Part model, mm, in its own coordinate system. Give positions to 0.01 mm unless a question says otherwise; leave off trailing zeros.
1. Slice it at A-A on y = -1.9. Give the number of separate pieces and of enclosed holes in the cut face, and give its area (3 significant figures).
2. Probe line 1 (Z direction, x = 42, y = -2.9); line 2 (Z direction, x = -129, y = -0.95); line 3 (X direction, y = -2.25, z = -5.5). List the from-to ranges inside material, lowest first.
3. Drop flat-ended pins along their axis: pin 1 Ø2.5 at (x, z) = (-88, 1) entering from -Y; pin 2 Ø1 at (y, z) = (-2.5, -1.5) entering from +X. Give the stop position or say it passes through.
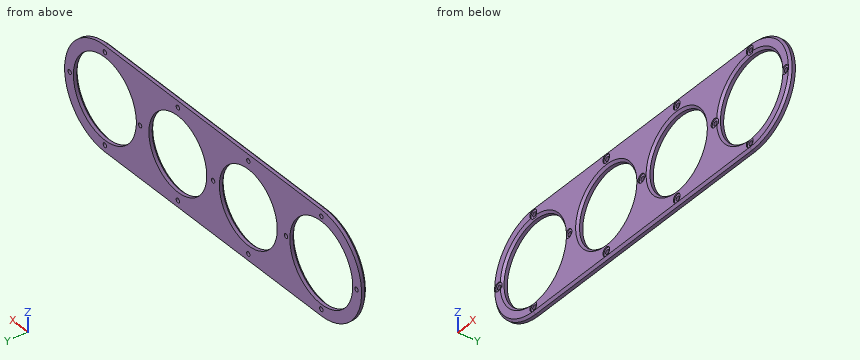
from build123d import *

# Parameters (mm, degrees)
F0_R     = 2
F0_R_2   = 37.5
F0_R_3   = 34.5
F1_DEPTH = 5
F2_SIZE  = 2
F3_SIZE  = 2
F4_R     = 4
F5_DEPTH = 1
F6_SIZE  = 1.99999


# Not quite as in the source:
# - a fillet or chamfer is up to 0.001 mm smaller than in the source, because OpenCascade refuses the exact size


with BuildPart() as f1:
    # F0 (on Front) → F1 (new body)
    with BuildSketch(Plane.XZ):
        with BuildLine():
            ThreePointArc((129, -48), (177, 0), (129, 48))
            Line((129, 48), (0, 48))
            Line((0, 48), (-129, 48))
            ThreePointArc((-129, 48), (-177, 0), (-129, -48))
            Line((-129, -48), (0, -48))
            Line((0, -48), (129, -48))
        make_face()
        with Locations((-129, -42)):
            Circle(F0_R, mode=Mode.SUBTRACT)
        with Locations((-42, -42)):
            Circle(F0_R, mode=Mode.SUBTRACT)
        with Locations((42, -42)):
            Circle(F0_R, mode=Mode.SUBTRACT)
        with Locations((129, -42)):
            Circle(F0_R, mode=Mode.SUBTRACT)
        with Locations((-171, 0)):
            Circle(F0_R, mode=Mode.SUBTRACT)
        with Locations((-129, 0)):
            Circle(F0_R_2, mode=Mode.SUBTRACT)
        with Locations((-87, 0)):
            Circle(F0_R, mode=Mode.SUBTRACT)
        with Locations((-42, 0)):
            Circle(F0_R_3, mode=Mode.SUBTRACT)
        with Locations((-129, 42)):
            Circle(F0_R, mode=Mode.SUBTRACT)
        with Locations((-42, 42)):
            Circle(F0_R, mode=Mode.SUBTRACT)
        Circle(F0_R, mode=Mode.SUBTRACT)
        with Locations((42, 0)):
            Circle(F0_R_3, mode=Mode.SUBTRACT)
        with Locations((87, 0)):
            Circle(F0_R, mode=Mode.SUBTRACT)
        with Locations((129, 0)):
            Circle(F0_R_2, mode=Mode.SUBTRACT)
        with Locations((171, 0)):
            Circle(F0_R, mode=Mode.SUBTRACT)
        with Locations((42, 42)):
            Circle(F0_R, mode=Mode.SUBTRACT)
        with Locations((129, 42)):
            Circle(F0_R, mode=Mode.SUBTRACT)
    extrude(amount=F1_DEPTH)

    # F2
    f2_edges = [f1.edges().sort_by_distance(p)[0] for p in [
        (7.5, -5, 0),
        (-76.5, -5, 0),
    ]]
    chamfer(f2_edges, length=F2_SIZE)

    # F3
    f3_edges = [f1.edges().sort_by_distance(p)[0] for p in [
        (91.5, -5, 0),
        (-166.5, -5, 0),
    ]]
    chamfer(f3_edges, length=F3_SIZE)

    # F4 (on face) → F5 (cut)
    with BuildSketch(Plane.XZ.offset(5)):
        Circle(F4_R)
        with Locations((42, 42)):
            Circle(F4_R)
        with Locations((42, -42)):
            Circle(F4_R)
        with Locations((129, 42)):
            Circle(F4_R)
        with Locations((87, 0)):
            Circle(F4_R)
        with Locations((129, -42)):
            Circle(F4_R)
        with Locations((171, 0)):
            Circle(F4_R)
        with Locations((-42, 42)):
            Circle(F4_R)
        with Locations((-42, -42)):
            Circle(F4_R)
        with Locations((-87, 0)):
            Circle(F4_R)
        with Locations((-129, -42)):
            Circle(F4_R)
        with Locations((-129, 42)):
            Circle(F4_R)
        with Locations((-171, 0)):
            Circle(F4_R)
    extrude(amount=-F5_DEPTH, mode=Mode.SUBTRACT)

    # F6 (size 2 in the source; OpenCascade refuses exactly that, so slightly less here)
    f6_edges = [f1.edges().sort_by_distance(p)[0] for p in [
        (-177, -5, 0),
        (0, -5, 48),
        (0, -5, -48),
        (177, -5, 0),
    ]]
    chamfer(f6_edges, length=F6_SIZE)


solid = f1.part
Data:
1. separate pieces: 1
1. enclosed holes: 17
1. area: 15,500 mm2
2. line 1: z = -48 to -44, -40 to -34.5, 34.5 to 40, 44 to 48
2. line 2: z = -48 to -44, -40 to -37.5, 37.5 to 40, 44 to 48
2. line 3: x = -176.68 to -166.09, -91.91 to -76.06, -7.94 to 7.94, 76.06 to 91.91, 166.09 to 176.68
3. pin 1: stops at y = -4
3. pin 2: stops at x = 176.99
